Design review of the part built by this model. Coordinates are the model's own, in mm. Face numbers are marked on the shaded views. A direction names the side the tool comes from. Give positions to 0.01 mm unless a question says otherwise; leave off trailing zeros. Write each loop counter-clockwise with the first axis right and the second up, starting at its lowest first coordinate (ties: lowest second). Pieces come first, ordered by that corner, then holes. Notation, with made-up numbers: (63, 77) - (122, 77) arc R18 cw to (122, 105) - close; hole circle Ø5 at (65.5, -8). An arc over 180 degrees is marked (long way). Use a Markdown table: item, result. Add a question column.
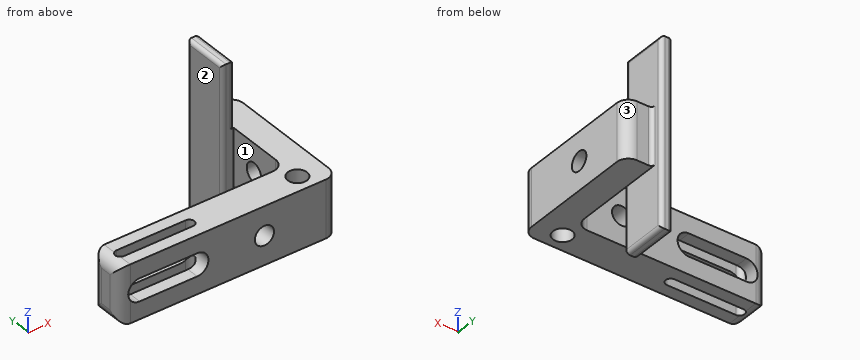
```python
from build123d import *

# Parameters (mm, degrees)
BOSS_EXTRUDE1_DEPTH = 15
CUT_EXTRUDE1_DEPTH  = 69.805886376
CUT_EXTRUDE2_DEPTH  = 69.805886376
SKETCH4_W           = 49
SKETCH4_H           = 12
BOSS_EXTRUDE2_DEPTH = 3
SKETCH5_R           = 2.5
CUT_EXTRUDE3_DEPTH  = 76.863364017
FILLET1_R           = 3
FILLET2_R           = 3
FILLET3_R           = 1
FILLET4_R           = 3
FILLET5_R           = 1
SKETCH6_R           = 2.5
CUT_EXTRUDE4_DEPTH  = 71.754858561
SKETCH7_R           = 2.5
CUT_EXTRUDE5_DEPTH  = 72.716455573


with BuildPart() as part:
    # Sketch1 → Boss-Extrude1 (new body)
    with BuildSketch(Plane.XY):
        Polygon((0, 0), (57, 0), (57, 35.5), (50, 35.5), (50, 9), (0, 9), align=None)
    extrude(amount=-BOSS_EXTRUDE1_DEPTH)

    # Sketch2 → Cut-Extrude1 (cut, through all)
    with BuildSketch(Plane.XZ):
        with BuildLine():
            Line((5.45, -4.55), (20.45, -4.55))
            ThreePointArc((20.45, -4.55), (23.4, -7.5), (20.45, -10.45))
            Line((20.45, -10.45), (5.45, -10.45))
            ThreePointArc((5.45, -10.45), (2.5, -7.5), (5.45, -4.55))
        make_face()
    extrude(amount=-CUT_EXTRUDE1_DEPTH, mode=Mode.SUBTRACT)

    # Sketch3 → Cut-Extrude2 (cut, through all)
    with BuildSketch(Plane.XY):
        with BuildLine():
            Line((3.8, 5.8), (21.8, 5.8))
            ThreePointArc((21.8, 5.8), (23.1, 4.5), (21.8, 3.2))
            Line((21.8, 3.2), (3.8, 3.2))
            ThreePointArc((3.8, 3.2), (2.5, 4.5), (3.8, 5.8))
        make_face()
    extrude(amount=-CUT_EXTRUDE2_DEPTH, mode=Mode.SUBTRACT)

    # Sketch4 → Boss-Extrude2 (add)
    with BuildSketch(Plane.ZY.offset(-50)):
        with Locations((-7.5, 32.5)):
            Rectangle(SKETCH4_W, SKETCH4_H)
    extrude(amount=BOSS_EXTRUDE2_DEPTH)

    # Sketch5 → Cut-Extrude3 (cut, through all)
    with BuildSketch(Plane.XY):
        with Locations((50, 4.5)):
            Circle(SKETCH5_R)
    extrude(amount=-CUT_EXTRUDE3_DEPTH, mode=Mode.SUBTRACT)

    # Fillet1
    fillet1_edges = [part.edges().sort_by_distance(p)[0] for p in [
        (50, 9, -7.5),
        (57, 0, -7.5),
    ]]
    fillet(fillet1_edges, radius=FILLET1_R)

    # Fillet2
    # the kernel refuses this fillet: 3 mm, written as the material it takes off along each edge
    with BuildSketch(Plane(origin=(0, 9, 7.5), x_dir=(0, -1, 0), z_dir=(0, 0, -1)), Plane(origin=(0, 0, 7.5), x_dir=(1, 0, 0), z_dir=(0, 0, -1))) as fillet2_piece_1:
        with BuildLine():
            CenterArc((FILLET2_R, -FILLET2_R), FILLET2_R, 90, 90)
            Line((0, -FILLET2_R), (0, 0))
            Line((0, 0), (FILLET2_R, 0))
        make_face()
    extrude(amount=30, mode=Mode.SUBTRACT)
    with BuildSketch(Plane(origin=(0, 16.5, -15), x_dir=(0, 0, 1), z_dir=(0, -1, 0)), Plane(origin=(0, 16.5, 0), x_dir=(1, 0, 0), z_dir=(0, -1, 0))) as fillet2_piece_2:
        with BuildLine():
            CenterArc((FILLET2_R, -FILLET2_R), FILLET2_R, 90, 90)
            Line((0, -FILLET2_R), (0, 0))
            Line((0, 0), (FILLET2_R, 0))
        make_face()
    extrude(amount=24, mode=Mode.SUBTRACT)

    # Fillet3
    fillet3_edges = [part.edges().sort_by_distance(p)[0] for p in [
        (50, 26.5, 8.5),
        (50, 32.5, -32),
        (50, 38.5, -7.5),
        (50, 32.5, 17),
        (47, 32.5, -32),
        (47, 32.5, 17),
        (47, 26.5, -7.5),
        (47, 38.5, -7.5),
    ]]
    fillet(fillet3_edges, radius=FILLET3_R)

    # Fillet4
    fillet4_edges = [part.edges().sort_by_distance(p)[0] for p in [
        (57, 35.5, -7.5),
    ]]
    fillet(fillet4_edges, radius=FILLET4_R)

    # Fillet5
    fillet5_edges = [part.edges().sort_by_distance(p)[0] for p in [
        (50, 35.5, -7.5),
    ]]
    fillet(fillet5_edges, radius=FILLET5_R)

    # Sketch6 → Cut-Extrude4 (cut, through all)
    with BuildSketch(Plane.ZY.offset(-50)):
        with Locations((-7.5, 19.488510255)):
            Circle(SKETCH6_R)
    extrude(amount=-CUT_EXTRUDE4_DEPTH, mode=Mode.SUBTRACT)

    # Sketch7 → Cut-Extrude5 (cut, through all)
    with BuildSketch(Plane(origin=(0, 9, 0), x_dir=(1, 0, 0), z_dir=(0, 1, 0))):
        with Locations(Location((38, 7.5, 0), (0, 0, 180))):
            Circle(SKETCH7_R)
    extrude(amount=-CUT_EXTRUDE5_DEPTH, mode=Mode.SUBTRACT)


solid = part.part
```
(1) For line 1 along Z through (x, y) = (38, 4); line 2 along Z through (x, y) = (31, 4.5); line 3 along X through (y, z) = (32, 9), list the stretches that pass through material, from the lowest coordinate up.
(2) Add section A-A (x = 7.5). State the section outline as (y, z) points, and give its area (3 significant figures).
(3) Insertion check: pin 1 (11 mm diameter, centred on y = 32, z = -15, fed in from -X); pin 2 (4 mm diameter, centred on x = 50, y = 4.5, fed in from +Z); pin 3 (2.5 mm diameter, centred on x = 12.5, y = 2, fed in from -Z); pin 4 (1 mm diameter, centred on x = 14.5, y = 1, fed in from +Z). Each pin has a flat end and moves straight along its axis. Give the tip position at first contact, or say it passes through.
(4) Add section C-C (y = 25.5). State the section outline as (x, z) points.
(5) Add section B-B (z = 5.5). State the section outline as (x, y) points.
(6) Add section D-D (z = -13). State the section outline as (x, y) points.
(7) Tool access review of the marked faces 1, 2 and 3: name each direction out of +Z, -Z, +X, -X, +Y, -Y from which nothing blocks a thin tool from reaching the whole face with its end or side.
Answers follow:
| question | item | result |
|---|---|---|
| 1 | line 1 | -15 to -10, -5 to 0 |
| 1 | line 2 | -15 to 0 |
| 1 | line 3 | 47 to 50 |
| 2 | outline | (0, -15) - (3.2, -15) - (3.2, -10.45) - (0, -10.45) - close; (0, -4.55) - (3.2, -4.55) - (3.2, 0) - (0, 0) - close; (5.8, -15) - (9, -15) - (9, -10.45) - (5.8, -10.45) - close; (5.8, -4.55) - (9, -4.55) - (9, 0) - (5.8, 0) - close |
| 2 | area | 58.2 mm^2 |
| 3 | pin 1 | x = 47 |
| 3 | pin 2 | through |
| 3 | pin 3 | z = -15 |
| 3 | pin 4 | z = 0 |
| 4 | outline | (50, -15) - (57, -15) - (57, 0) - (50, 0) - close |
| 5 | outline | (47, 27.5) arc R1 ccw to (48, 26.5) - (49, 26.5) arc R1 ccw to (50, 27.5) - (50, 37.5) arc R1 ccw to (49, 38.5) - (48, 38.5) arc R1 ccw to (47, 37.5) - close |
| 6 | outline | (0.17, 2) arc R3 ccw to (3, 0) - (54, 0) arc R3 ccw to (57, 3) - (57, 32.5) arc R3 ccw to (54, 35.5) - (51, 35.5) arc R1 cw to (50, 36.5) - (50, 37.5) arc R1 ccw to (49, 38.5) - (48, 38.5) arc R1 ccw to (47, 37.5) - (47, 27.5) arc R1 ccw to (48, 26.5) - (50, 26.5) - (50, 12) arc R3 cw to (47, 9) - (3, 9) arc R3 ccw to (0.17, 7) - close; hole (3.8, 3.2) - (21.8, 3.2) arc R1.3 ccw to (21.8, 5.8) - (3.8, 5.8) arc R1.3 ccw to start; hole circle Ø5 at (50, 4.5) |
| 7 | face 1 | +Z, -Z, -X |
| 7 | face 2 | +Z, -Z, -X, +Y |
| 7 | face 3 | +Z, -Z, +X, +Y |
